Answer from the drawing. Dimensions are ordinates in mm from the lowest x, y and z of the part. Coordinates: 2 decimals unless noted, no trailing zeros. Write each loop counter-clockwise with the first axis right and the second up, starting at its lowest first coordinate (ties: lowest second). Pieces come first, ordered by that corner, then holes.
(1) Straight lines are drawn through the part: line 1 (X direction, y = 4.25, z = 53); line 2 (Z direction, x = 125, y = 2.25); line 3 (Z direction, x = 6.5, y = 3.5). For each, find the intervals that lie inside material, in ascending order.
(2) The part is cut by section C-C on y = 1.5. Give the number of separate pieces and of enclosed holes in the cut face, plus the area to 3 significant figures.
(3) The part is cut by section B-B on x = 38. Determine the outline of the cut face in (y, z), plus the area to 3 significant figures.
(4) Given P1, Ø3.5, axis at x = 125, z = 53, coming from the +Y side; P2, Ø3, axis at y = 1.5, z = 30, coming from the -X side; P3, Ø1.5, axis at x = 29, y = 2, coming from the -Z side, each flat-ended and moving along its own axis, determine where each tip first touches the part or whether it passes through.
(5) The part is cut by section D-D on x = 9. Determine the outline of the cut face in (y, z), plus the area to 3 significant figures.
(6) The part is cut by section A-A on z = 103. Determine the outline of the cut face in (x, y).
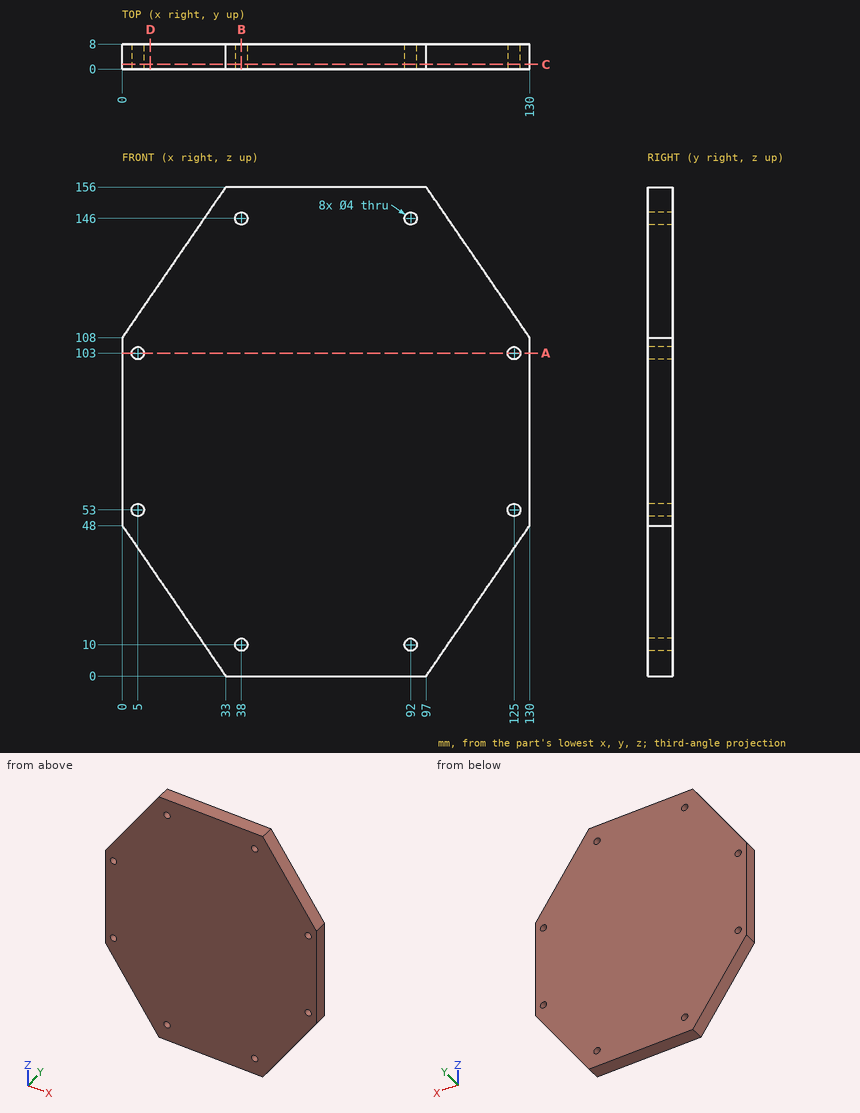
Model answer:
1. line 1: x = 0 to 3, 7 to 123, 127 to 130
1. line 2: z = 40.73 to 51, 55 to 101, 105 to 115.27
1. line 3: z = 38.55 to 51.68, 54.32 to 101.68, 104.32 to 117.45
2. separate pieces: 1
2. enclosed holes: 8
2. area: 17,000 mm2
3. outline: (0, 0) - (8, 0) - (8, 8) - (0, 8) - close; (0, 12) - (8, 12) - (8, 144) - (0, 144) - close; (0, 148) - (8, 148) - (8, 156) - (0, 156) - close
3. area: 1,180 mm2
4. P1: passes through
4. P2: stops at x = 11.34
4. P3: stops at z = 4.73
5. outline: (0, 34.91) - (8, 34.91) - (8, 121.09) - (0, 121.09) - close
5. area: 689 mm2
6. outline: (0, 0) - (3, 0) - (3, 8) - (0, 8) - close; (7, 0) - (123, 0) - (123, 8) - (7, 8) - close; (127, 0) - (130, 0) - (130, 8) - (127, 8) - close
